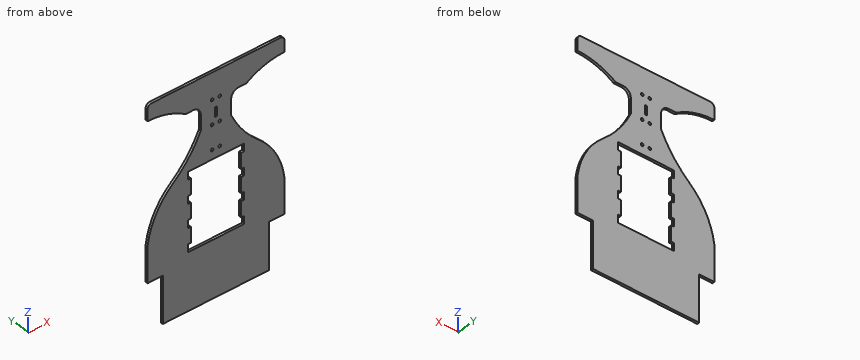
Autodesk Inventor part; units mm, degrees
ref_plane "YZ Plane" through (0, 0, 0) normal (1, 0, 0) x (0, 1, 0)
ref_plane "XZ Plane" through (0, 0, 0) normal (0, 1, 0) x (-1, 0, 0)
ref_plane "XY Plane" through (0, 0, 0) normal (0, 0, 1) x (1, 0, 0)
sketch "草圖1" plane through (0, 0, 0) normal (0, 1, 0) x (-1, 0, 0)
  line L0 (413.5961, 122.1998) -> (413.5961, 137.1998)
  arc A0 (413.5961, 137.1998) -> (408.5961, 142.1998) centre (408.5961, 137.1998) ccw
  line L1 (233.5961, 122.1998) -> (233.5961, 137.1998)
  line L2 (238.5961, 142.1998) -> (408.5961, 142.1998)
  line L3 (303.5961, 77.1998) -> (303.5961, 97.1998)
  arc A1 (303.5961, 97.1998) -> (293.5961, 107.1998) centre (293.5961, 97.1998) ccw
  line L4 (293.5961, 107.1998) -> (283.5961, 107.1998)
  line L5 (343.5961, 77.1998) -> (343.5961, 97.1998)
  arc A2 (353.5961, 107.1998) -> (343.5961, 97.1998) centre (353.5961, 97.1998) ccw
  line L6 (353.5961, 107.1998) -> (363.5961, 107.1998)
  line L7 (233.5961, 137.1998) -> (233.5961, 122.1998)
  arc A3 (238.5961, 142.1998) -> (233.5961, 137.1998) centre (238.5961, 137.1998) ccw
  arc A4 (283.5961, 107.1998) -> (233.5961, 122.1998) centre (233.5961, 31.3665) ccw
  arc A5 (413.5961, 122.1998) -> (363.5961, 107.1998) centre (413.5961, 31.3665) ccw
  line L8 (356.5961, 34.1998) -> (290.5961, 34.1998)
  line L9 (290.5961, 24.1998) -> (290.5961, 4.1998)
  line L10 (290.5961, -5.8002) -> (290.5961, -25.8002)
  line L11 (290.5961, -35.8002) -> (290.5961, -55.8002)
  line L12 (290.5961, -65.8002) -> (356.5961, -65.8002)
  line L13 (263.5961, -138.8002) -> (383.5961, -138.8002)
  line L14 (233.6991, -53.0551) -> (233.6991, -78.8002)
  line L15 (413.5961, -78.8002) -> (413.4932, -53.0551)
  arc A6 (267.2809, 29.4379) -> (303.5961, 77.1998) centre (176.7496, 135.9594) ccw
  arc A7 (267.2809, 29.4379) -> (233.6991, -32.0184) centre (330.5999, -45.0649) ccw
  arc A8 (343.5961, 77.1998) -> (379.9114, 29.4379) centre (470.4427, 135.9594) ccw
  arc A9 (413.4932, -32.0184) -> (379.9114, 29.4379) centre (316.5923, -45.0649) ccw
  line L16 (413.4932, -32.0184) -> (413.4932, -53.0551)
  line L17 (233.6991, -32.0184) -> (233.6991, -53.0551)
  line L18 (290.5961, -55.8002) -> (290.5961, -35.8002)
  line L19 (290.5961, -25.8002) -> (290.5961, -5.8002)
  line L20 (290.5961, 4.1998) -> (290.5961, 24.1998)
  line L21 (290.5961, 34.1998) -> (287.5961, 34.1998)
  line L22 (287.5961, -65.8002) -> (290.5961, -65.8002)
  line L23 (287.5961, 4.1998) -> (290.5961, 4.1998)
  line L24 (290.5961, 4.1998) -> (290.5961, 24.1998)
  line L25 (290.5961, 24.1998) -> (287.5961, 24.1998)
  line L26 (290.5961, -5.8002) -> (287.5961, -5.8002)
  line L27 (287.5961, -25.8002) -> (290.5961, -25.8002)
  line L28 (290.5961, -25.8002) -> (290.5961, -5.8002)
  line L29 (290.5961, -35.8002) -> (287.5961, -35.8002)
  line L30 (287.5961, -55.8002) -> (290.5961, -55.8002)
  line L31 (290.5961, -55.8002) -> (290.5961, -35.8002)
  line L32 (287.5961, 34.1998) -> (286.5961, 34.1998)
  line L33 (286.5961, 34.1998) -> (286.5961, 24.1998)
  line L34 (286.5961, 4.1998) -> (286.5961, -5.8002)
  line L35 (286.5961, -25.8002) -> (286.5961, -35.8002)
  line L36 (286.5961, -55.8002) -> (286.5961, -65.8002)
  line L37 (286.5961, -65.8002) -> (287.5961, -65.8002)
  line L38 (287.5961, 24.1998) -> (286.5961, 24.1998)
  line L39 (287.5961, 4.1998) -> (286.5961, 4.1998)
  line L40 (287.5961, -5.8002) -> (286.5961, -5.8002)
  line L41 (287.5961, -25.8002) -> (286.5961, -25.8002)
  line L42 (287.5961, -35.8002) -> (286.5961, -35.8002)
  line L43 (287.5961, -55.8002) -> (286.5961, -55.8002)
  line L44 (356.5961, 24.1998) -> (356.5961, 4.1998)
  line L45 (356.5961, -5.8002) -> (356.5961, -25.8002)
  line L46 (356.5961, -35.8002) -> (356.5961, -55.8002)
  line L47 (356.5961, -55.8002) -> (356.5961, -35.8002)
  line L48 (356.5961, -25.8002) -> (356.5961, -5.8002)
  line L49 (356.5961, 4.1998) -> (356.5961, 24.1998)
  line L50 (356.5961, 34.1998) -> (359.5961, 34.1998)
  line L51 (359.5961, -65.8002) -> (356.5961, -65.8002)
  line L52 (359.5961, 4.1998) -> (356.5961, 4.1998)
  line L53 (356.5961, 4.1998) -> (356.5961, 24.1998)
  line L54 (356.5961, 24.1998) -> (359.5961, 24.1998)
  line L55 (356.5961, -5.8002) -> (359.5961, -5.8002)
  line L56 (359.5961, -25.8002) -> (356.5961, -25.8002)
  line L57 (356.5961, -25.8002) -> (356.5961, -5.8002)
  line L58 (356.5961, -35.8002) -> (359.5961, -35.8002)
  line L59 (359.5961, -55.8002) -> (356.5961, -55.8002)
  line L60 (356.5961, -55.8002) -> (356.5961, -35.8002)
  line L61 (359.5961, 34.1998) -> (360.5961, 34.1998)
  line L62 (360.5961, 34.1998) -> (360.5961, 24.1998)
  line L63 (360.5961, 4.1998) -> (360.5961, -5.8002)
  line L64 (360.5961, -25.8002) -> (360.5961, -35.8002)
  line L65 (360.5961, -55.8002) -> (360.5961, -65.8002)
  line L66 (360.5961, -65.8002) -> (359.5961, -65.8002)
  line L67 (359.5961, 24.1998) -> (360.5961, 24.1998)
  line L68 (359.5961, 4.1998) -> (360.5961, 4.1998)
  line L69 (359.5961, -5.8002) -> (360.5961, -5.8002)
  line L70 (359.5961, -25.8002) -> (360.5961, -25.8002)
  line L71 (359.5961, -35.8002) -> (360.5961, -35.8002)
  line L72 (359.5961, -55.8002) -> (360.5961, -55.8002)
  line L73 (323.5961, 97.1998) -> (325.0961, 97.1998)
  line L74 (325.0961, 97.1998) -> (325.0961, 89.1998)
  line L75 (325.0961, 85.1998) -> (322.0961, 85.1998)
  line L76 (322.0961, 89.1998) -> (322.0961, 97.1998)
  line L77 (322.0961, 97.1998) -> (323.5961, 97.1998)
  line L78 (322.0961, 85.1998) -> (322.0961, 89.1998)
  line L79 (325.0961, 85.1998) -> (325.0961, 89.1998)
  line L80 (323.5961, 77.1998) -> (408.5961, 77.1998) construction
  line L81 (323.5961, 77.1998) -> (238.5961, 77.1998) construction
  line L82 (408.5961, 107.1998) -> (393.5961, 107.1998) construction
  line L83 (393.5961, 107.1998) -> (393.5961, 47.1998) construction
  line L84 (393.5961, 47.1998) -> (423.5961, 47.1998) construction
  line L85 (423.5961, 47.1998) -> (423.5961, 107.1998) construction
  line L86 (423.5961, 107.1998) -> (408.5961, 107.1998) construction
  line L87 (238.5961, 107.1998) -> (253.5961, 107.1998) construction
  line L88 (253.5961, 107.1998) -> (253.5961, 47.1998) construction
  line L89 (253.5961, 47.1998) -> (223.5961, 47.1998) construction
  line L90 (223.5961, 47.1998) -> (223.5961, 107.1998) construction
  line L91 (223.5961, 107.1998) -> (238.5961, 107.1998) construction
  line L92 (253.5961, 77.1998) -> (257.5961, 77.1998) construction
  line L93 (257.5961, 77.1998) -> (257.5961, 82.1998) construction
  line L94 (393.5961, 77.1998) -> (389.5961, 77.1998) construction
  line L95 (389.5961, 77.1998) -> (389.5961, 82.1998) construction
  line L96 (257.5961, 77.1998) -> (261.5961, 77.1998) construction
  line L97 (389.5961, 77.1998) -> (385.5961, 77.1998)
  line L98 (261.5961, 77.1998) -> (271.5961, 77.1998)
  line L99 (271.5961, 77.1998) -> (318.5808, 60.0988) construction
  line L100 (271.5961, 77.1998) -> (318.5808, 94.3008) construction
  line L101 (385.5961, 77.1998) -> (375.5961, 77.1998)
  line L102 (375.5961, 77.1998) -> (328.6115, 94.3008) construction
  line L103 (375.5961, 77.1998) -> (328.6115, 60.0988) construction
  line L104 (261.5961, 77.1998) -> (274.2452, 39.2525) construction
  line L105 (274.2452, 39.2525) -> (372.947, 39.2525) construction
  line L106 (372.947, 39.2525) -> (385.5961, 77.1998) construction
  line L107 (323.5961, -108.8002) -> (408.5961, -108.8002) construction
  line L108 (323.5961, -108.8002) -> (238.5961, -108.8002) construction
  line L109 (423.5961, -108.8002) -> (423.5961, -78.8002) construction
  line L110 (423.5961, -78.8002) -> (393.5961, -78.8002)
  line L111 (393.5961, -78.8002) -> (393.5961, -138.8002)
  line L112 (393.5961, -138.8002) -> (423.5961, -138.8002) construction
  line L113 (423.5961, -138.8002) -> (423.5961, -108.8002) construction
  line L114 (223.5961, -108.8002) -> (223.5961, -78.8002) construction
  line L115 (223.5961, -78.8002) -> (253.5961, -78.8002)
  line L116 (253.5961, -78.8002) -> (253.5961, -138.8002)
  line L117 (253.5961, -138.8002) -> (223.5961, -138.8002) construction
  line L118 (223.5961, -138.8002) -> (223.5961, -108.8002) construction
  line L119 (393.5961, -138.8002) -> (383.5961, -138.8002)
  line L120 (263.5961, -138.8002) -> (253.5961, -138.8002)
  line L121 (318.5808, 94.3008) -> (318.5808, 108.3008) construction
  line L122 (328.6115, 94.3008) -> (328.6115, 108.3008) construction
  line L123 (328.6115, 60.0988) -> (328.6115, 46.0988) construction
  line L124 (318.5808, 60.0988) -> (318.5808, 46.0988) construction
  circle A10 centre (328.6115, 108.3008) radius 1.8
  circle A11 centre (318.5808, 108.3008) radius 1.8
  circle A12 centre (328.6115, 46.0988) radius 1.8
  circle A13 centre (318.5808, 46.0988) radius 1.8
  circle A14 centre (318.5808, 77.1998) radius 1.8
  circle A15 centre (328.6115, 77.1998) radius 1.8
  point P0 (0, 0)
  dimension "d0" = 14
  dimension "d1" = 14
  dimension "d2" = 14
  dimension "d3" = 3.6
  dimension "d4" = 3.6
  dimension "d5" = 3.6
  dimension "d6" = 3.6
  dimension "d7" = 3.6
  dimension "d8" = 3.6
extrude "擠出1" add sketch "草圖1" along normal blind 3
ref_plane "Work Plane1" through (-323.5961, 0, 97.1998) normal (1, 0, 0) x (0, 0, -1)
properties part number "底盤新"
Check sheet for the modelled part. Datum: model origin and axes. Units: mm. Round coordinates to 2 decimals unless told otherwise and drop trailing zeros. Write each loop counter-clockwise with the first axis right and the second up, starting at its lowest first coordinate (ties: lowest second). Pieces come first, ordered by that corner, then holes. Notation, with made-up numbers: (27, 79.25) -> (47, 79.25) arc R20 cw to (47, 104.25) -> close; hole circle Ø4 at (-28, 6). An arc over 180 degrees is marked (long way). One line per question, with ' | ' between items. Start each with the question number.
1. Sectioned sample at C-C, the plane z = -108.5. Record the cut outline in (x, y), then the cut area to 3 significant figures.
2. Scan lines: line 1 along X through (y, z) = (1.3, -39.5); line 2 along Z through (x, y) = (-298, 2.3); line 3 along Z through (x, y) = (-288, 1.15). Record each from-to range of solid material in increasing order. Write a range as from..to.
3. Sectioned sample at D-D, the plane y = 0.55. Count the separate pieces of the cut face and the enclosed holes in it, then the cut area to 3 significant figures.
4. Sectioned sample at B-B, the plane x = -279. Record the cut outline in (y, z), then the cut area to 3 significant figures.
5. Depth check by flat-ended pin: pin 1 (4 mm diameter, centred on x = -318.58, z = 46.1, fed in from -Y); pin 2 (1.5 mm diameter, centred on y = 1.5, z = 31, fed in from -X); pin 3 (0.9 mm diameter, centred on y = 2, z = 84.5, fed in from +X). Enter the tip coordinate at first touch or a pass-through.
6. Sectioned sample at A-A, the plane x = -309. Record the cut outline in (y, z), then the cut area to 3 significant figures.
Taken from the geometry:
1) outline: (-393.6, 0) -> (-253.6, 0) -> (-253.6, 3) -> (-393.6, 3) -> close | area: 420 mm^2
2) line 1: x = -413.49..-356.6, -290.6..-233.7 | line 2: z = -138.8..-65.8, 34.2..66.38, 106.18..142.2 | line 3: z = -138.8..-65.8, -55.8..-35.8, -25.8..-5.8, 4.2..24.2, 34.2..51.31, 107.2..142.2
3) separate pieces: 1 | enclosed holes: 8 | area: 29,300 mm^2
4) outline: (0, -138.8) -> (3, -138.8) -> (3, 40.63) -> (0, 40.63) -> close; (0, 110.04) -> (3, 110.04) -> (3, 142.2) -> (0, 142.2) -> close | area: 635 mm^2
5) pin 1: stops at y = 0 | pin 2: stops at x = -378.96 | pin 3: stops at x = -303.6
6) outline: (0, -138.8) -> (3, -138.8) -> (3, -65.8) -> (0, -65.8) -> close; (0, 34.2) -> (3, 34.2) -> (3, 142.2) -> (0, 142.2) -> close | area: 543 mm^2
